Can you work these out from the model? Positions are in its coordinate system, mm. A direction names the side the tool comes from. Give positions to 0.01 mm unless a question says otherwise; leave off trailing zeros. Order: outer loops, then holes, each group sorted by start corner. A loop starts at its lowest first (then second) coordinate and runs counter-clockwise, first axis right, second up.
```python
from build123d import *

# Parameters (mm, degrees)
F0_R     = 21.5
F0_W     = 10
F0_H     = 6.020403
F1_DEPTH = 2.5


with BuildPart() as f1:
    # F0 (on Top) → F1 (new body)
    with BuildSketch(Plane.XY):
        Circle(F0_R)
        with Locations((-10.591081, -5.972431)):
            Rectangle(F0_W, F0_H, mode=Mode.SUBTRACT)
        with Locations((10.591081, -5.972431)):
            Rectangle(F0_W, F0_H, mode=Mode.SUBTRACT)
        with Locations((-10.591081, 5.972431)):
            Rectangle(F0_W, F0_H, mode=Mode.SUBTRACT)
        with Locations((10.591081, 5.972431)):
            Rectangle(F0_W, F0_H, mode=Mode.SUBTRACT)
    extrude(amount=F1_DEPTH)


solid = f1.part
```
1) Which directions (+Z, -Z, +X, -X, +Y, -Y) give clear straight access to the entire face, cutting with the end or side of a thin tool? Please do faces 1 (the face through (-11, -2.962, 1)), 2 (the face through (0, 0, 0)).
2) Suppose I cut it at B-B (z = 1.85). Please give me the cut outline in (x, y).
3) We'd pull the mould along X, two halves only. Please class faces 3 (the face through (0, 0, 2.5)), 4 (the face through (11, -8.983, 1)), 5 (the face through (-2.799, 21.317, 1.232)): +X half, -X half, draft (parallel to the pull), parting line (faces both ways), or undercut.
4) Suppose I cut it at A-A (x = 15). Please give me the cut outline in (y, z).
5) Suppose I cut it at C-C (y = -5.5). Please give me the cut outline in (x, z).
6) If I drill on line 1 (X direction, y = 6, z = 1.6); line 2 (X direction, y = -3.5, z = 1.35); line 3 (Y direction, x = 12.5, z = 1.5), over which ranges is the centre line in solid material (lowest first)?
7) Suppose I cut it at D-D (y = -10). Please give me the cut outline in (x, z).
8) I'm going to push flat-ended pins straight in: pin 1 Ø0.8 at (y, z) = (7, 0.5) entering from +X; pin 2 Ø3 at (x, y) = (13.5, 8) entering from +Z; pin 3 Ø1.2 at (y, z) = (-5, 1.5) entering from +X; pin 4 Ø1 at (y, z) = (13, 1.5) entering from -X. Where does each tip first touch, or does it pass through?
Results:
1. face 1: +Z, -Z
1. face 2: -Z, +X, -X, +Y, -Y
2. outline: circle Ø43 at (0, 0); hole (-15.59, -8.98) - (-5.59, -8.98) - (-5.59, -2.96) - (-15.59, -2.96) - close; hole (-15.59, 2.96) - (-5.59, 2.96) - (-5.59, 8.98) - (-15.59, 8.98) - close; hole (5.59, -8.98) - (15.59, -8.98) - (15.59, -2.96) - (5.59, -2.96) - close; hole (5.59, 2.96) - (15.59, 2.96) - (15.59, 8.98) - (5.59, 8.98) - close
3. face 3: draft
3. face 4: undercut
3. face 5: parting line
4. outline: (-15.4, 0) - (-8.98, 0) - (-8.98, 2.5) - (-15.4, 2.5) - close; (-2.96, 0) - (2.96, 0) - (2.96, 2.5) - (-2.96, 2.5) - close; (8.98, 0) - (15.4, 0) - (15.4, 2.5) - (8.98, 2.5) - close
5. outline: (-20.78, 0) - (-15.59, 0) - (-15.59, 2.5) - (-20.78, 2.5) - close; (-5.59, 0) - (5.59, 0) - (5.59, 2.5) - (-5.59, 2.5) - close; (15.59, 0) - (20.78, 0) - (20.78, 2.5) - (15.59, 2.5) - close
6. line 1: x = -20.65 to -15.59, -5.59 to 5.59, 15.59 to 20.65
6. line 2: x = -21.21 to -15.59, -5.59 to 5.59, 15.59 to 21.21
6. line 3: y = -17.49 to -8.98, -2.96 to 2.96, 8.98 to 17.49
7. outline: (-19.03, 0) - (19.03, 0) - (19.03, 2.5) - (-19.03, 2.5) - close
8. pin 1: stops at x = 20.46
8. pin 2: stops at z = 2.5
8. pin 3: stops at x = 21.04
8. pin 4: stops at x = -17.49
